```python
from build123d import *

# Parameters (mm, degrees)
SKETCH_1_W          = 340
SKETCH_1_H          = 180
EXTRUDE_1_DEPTH     = 5
SKETCH_2_R          = 1.5
CUT_EXTRUDE_1_DEPTH = 5
SKETCH_4_R          = 4
CUT_EXTRUDE_2_DEPTH = 5


with BuildPart() as part:
    # 草图1 → 凸台-拉伸1 (new body)
    with BuildSketch(Plane(origin=(0, 0, 0), x_dir=(1, 0, 0), z_dir=(0, 1, 0))):
        with Locations((-170, 90)):
            Rectangle(SKETCH_1_W, SKETCH_1_H)
    extrude(amount=EXTRUDE_1_DEPTH)

    # 草图2 → 切除-拉伸1 (cut)
    with BuildSketch(Plane(origin=(0, 5, 0), x_dir=(1, 0, 0), z_dir=(0, 1, 0))):
        with Locations(Location((-330, 20, 0), (0, 0, 270))):
            Circle(SKETCH_2_R)
        with Locations(Location((-330, 40, 0), (0, 0, 270))):
            Circle(SKETCH_2_R)
        with Locations(Location((-330, 140, 0), (0, 0, 90))):
            Circle(SKETCH_2_R)
        with Locations(Location((-330, 160, 0), (0, 0, 90))):
            Circle(SKETCH_2_R)
        with Locations(Location((-10, 160, 0), (0, 0, 270))):
            Circle(SKETCH_2_R)
        with Locations(Location((-10, 140, 0), (0, 0, 270))):
            Circle(SKETCH_2_R)
        with Locations(Location((-10, 40, 0), (0, 0, 90))):
            Circle(SKETCH_2_R)
        with Locations(Location((-10, 20, 0), (0, 0, 90))):
            Circle(SKETCH_2_R)
    extrude(amount=-CUT_EXTRUDE_1_DEPTH, mode=Mode.SUBTRACT)

    # 草图4 → 切除-拉伸2 (cut)
    with BuildSketch(Plane(origin=(0, 5, 0), x_dir=(1, 0, 0), z_dir=(0, 1, 0))):
        with Locations(Location((-285, 140, 0), (0, 0, 270))):
            Circle(SKETCH_4_R)
        with Locations(Location((-285, 90, 0), (0, 0, 270))):
            Circle(SKETCH_4_R)
        with Locations(Location((-285, 40, 0), (0, 0, 270))):
            Circle(SKETCH_4_R)
        with Locations(Location((-55, 40, 0), (0, 0, 90))):
            Circle(SKETCH_4_R)
        with Locations(Location((-55, 90, 0), (0, 0, 90))):
            Circle(SKETCH_4_R)
        with Locations(Location((-55, 140, 0), (0, 0, 90))):
            Circle(SKETCH_4_R)
    extrude(amount=-CUT_EXTRUDE_2_DEPTH, mode=Mode.SUBTRACT)


solid = part.part
```
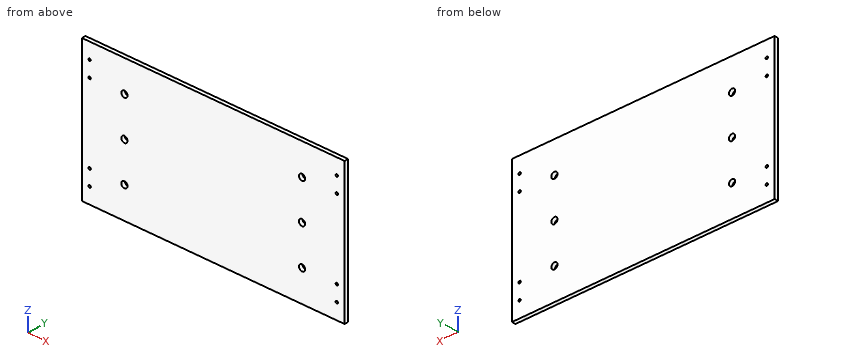
The listing builds one solid part. Answer for the finished solid, in the listing's coordinates (mm). Coordinates: 2 decimals unless noted, no trailing zeros. Loops run counter-clockwise (first coordinate to the right, second up) from the corner with the lowest first, then second, coordinate; pieces in that order, holes last. Notation, with made-up numbers: M 43.5,36.5 L 87.5,36.5 A13 ccw 87.5,43.5 Z; hole C -24,-5 d9. An arc over 180 degrees is marked long. Answer as CSV lines item,"result". Start each with the question number.
(1) The part is cut by section B-B (x = -55). Give the vertices of the cut face in (y, z), and give its area (3 significant figures).
(2) The part is cut by section A-A (z = -90). Give the vertices of the cut face in (x, y), and give its area (3 significant figures).
(3) Given pin 1 (2.5 mm diameter, centred on x = -10, z = -140, fed in from -Y), flat-ended and moving along its own axis, determine where the tip first touches the part or whether it passes through.
(4) Find the intervals of material crossed by L1, parallel to X at y = 1.2, z = -140; L2, parallel to X at y = 1.35, z = -160; L3, parallel to Z at x = -285, y = 2.1, in increasing order. Write a range as [from, to].
Determined:
1,outline,"M 0,-180 L 5,-180 L 5,-144 L 0,-144 Z; M 0,-136 L 5,-136 L 5,-94 L 0,-94 Z; M 0,-86 L 5,-86 L 5,-44 L 0,-44 Z; M 0,-36 L 5,-36 L 5,0 L 0,0 Z"
1,area,"780 mm2"
2,outline,"M -340,0 L -289,0 L -289,5 L -340,5 Z; M -281,0 L -59,0 L -59,5 L -281,5 Z; M -51,0 L 0,0 L 0,5 L -51,5 Z"
2,area,"1,620 mm2"
3,pin 1,"through"
4,L1,"[-340, -331.5], [-328.5, -289], [-281, -59], [-51, -11.5], [-8.5, 0]"
4,L2,"[-340, -331.5], [-328.5, -11.5], [-8.5, 0]"
4,L3,"[-180, -144], [-136, -94], [-86, -44], [-36, 0]"
